```python
from build123d import *

# Parameters (mm, degrees)
RESSALTO_EXTRUS_O1_DEPTH = 16
CORTE_EXTRUS_O1_DEPTH    = 32.953090617
ESBO_O8_W                = 3
ESBO_O8_H                = 20
CORTE_EXTRUS_O4_DEPTH    = 34.600595233
ESBO_O5_R                = 1
CORTE_EXTRUS_O2_DEPTH    = 5


with BuildPart() as part:
    # Esboço1 → Ressalto-extrusão1 (new body)
    with BuildSketch(Plane.XY):
        with BuildLine():
            Line((-6, 0), (-6, -27))
            Line((-6, -27), (6, -27))
            Line((6, -27), (6, 0))
            ThreePointArc((6, 0), (0, 6), (-6, 0))
        make_face()
    extrude(amount=RESSALTO_EXTRUS_O1_DEPTH)

    # Esboço2 → Corte-extrusão1 (cut, through all)
    with BuildSketch(Plane.XY.offset(16)):
        Polygon((0, 4.387862046), (-3.8, 2.193931023), (-3.8, -2.193931023), (0, -4.387862046), (3.8, -2.193931023), (3.8, 2.193931023), align=None)
    extrude(amount=-CORTE_EXTRUS_O1_DEPTH, mode=Mode.SUBTRACT)

    # Esboço8 → Corte-extrusão4 (cut, through all)
    with BuildSketch(Plane(origin=(6, 0, 0), x_dir=(0, 0, -1), z_dir=(1, 0, 0))):
        with Locations((-1.5, -17)):
            Rectangle(ESBO_O8_W, ESBO_O8_H)
    extrude(amount=-CORTE_EXTRUS_O4_DEPTH, mode=Mode.SUBTRACT)

    # Esboço5 → Corte-extrusão2 (cut)
    with BuildSketch(Plane.XZ.offset(27)):
        with Locations(Location((0, 13.5, 0), (0, 0, 270))):
            Circle(ESBO_O5_R)
        with Locations(Location((0, 5.5, 0), (0, 0, 270))):
            Circle(ESBO_O5_R)
    extrude(amount=-CORTE_EXTRUS_O2_DEPTH, mode=Mode.SUBTRACT)


solid = part.part
```
Check sheet for the modelled part. Datum: model origin and axes. Units: mm. A direction names the side the tool comes from. Coordinates: 2 decimals unless noted, no trailing zeros. Loops run counter-clockwise (first coordinate to the right, second up) from the corner with the lowest first, then second, coordinate; pieces in that order, holes last.
1) Gauge pin test, flat ends, axial feed: pin 1 (2 mm diameter, centred on x = 0, y = 1, fed in from -Z); pin 2 (0.9 mm diameter, centred on x = 1.5, z = 1.5, fed in from -Y); pin 3 (1 mm diameter, centred on x = 0, z = 13.5, fed in from -Y); pin 4 (1.5 mm diameter, centred on x = -2.5, z = 12, fed in from +Y). Record the tip position at first contact, or that the pin passes through.
2) Sectioned sample at B-B (x = -1.75). Record the boundary of the cut face in (y, z), and give its area (3 significant figures).
3) Release check for a two-part mould opening along X. For faces 4 (the face through (-6, -13, 10)), 5 (the face through (6, -14, 10)), 6 (the face through (1.87, -3.31, 8.11)), 7 (the face through (-1.927, -3.276, 8.112)) record: released by +X, released by -X, zero draft, split by the parting line, or undercut.
4) Sectioned sample at A-A (z = 11). Record the boundary of the cut face in (x, y), and give its area (3 significant figures).
5) Material ranges on probe 1 along X at (y, z) = (-25.3, 5.5); probe 2 along X at (y, z) = (-2, 15); probe 3 along Z at (x, y) = (3, -15), recorded low to high.
6) Sectioned sample at D-D (y = 3.5). Record the boundary of the cut face in (x, z).
7) Access from +Z, -Z, +X, -X, +Y, -Y to the whole of each face (thin tool, end or side, straight path). Record for faces 1 (the face through (0, -22, 14)), 2 (the face through (0, -17, 3)), 3 (the face through (-3.8, 0, 8)).
8) Sectioned sample at C-C (y = -24). Record the boundary of the cut face in (x, z).
Check sheet entries:
1. pin 1: passes through
1. pin 2: stops at y = -7
1. pin 3: stops at y = -22
1. pin 4: stops at y = 5.74
2. outline: (-27, 3) - (-7, 3) - (-7, 0) - (-3.38, 0) - (-3.38, 16) - (-27, 16) - close; (3.38, 0) - (5.74, 0) - (5.74, 16) - (3.38, 16) - close
2. area: 356 mm2
3. face 4: released by -X
3. face 5: released by +X
3. face 6: undercut
3. face 7: undercut
4. outline: (-6, -27) - (6, -27) - (6, 0) arc R6 ccw to (-6, 0) - close; hole (-3.8, -2.19) - (0, -4.39) - (3.8, -2.19) - (3.8, 2.19) - (0, 4.39) - (-3.8, 2.19) - close
4. area: 331 mm2
5. probe 1: x = -6 to -1, 1 to 6
5. probe 2: x = -6 to -3.8, 3.8 to 6
5. probe 3: z = 3 to 16
6. outline: (-4.87, 0) - (-1.54, 0) - (-1.54, 16) - (-4.87, 16) - close; (1.54, 0) - (4.87, 0) - (4.87, 16) - (1.54, 16) - close
7. face 1: -Y
7. face 2: -Z, +X, -X, -Y
7. face 3: +Z, -Z
8. outline: (-6, 3) - (6, 3) - (6, 16) - (-6, 16) - close; hole circle Ø2 at (0, 5.5); hole circle Ø2 at (0, 13.5)
